from build123d import *

# Parameters (mm, degrees)
F0_R     = 2.45
F0_W     = 1.981159
F0_H     = 1.5
F0_W_2   = 2.842553
F0_W_3   = 1.5
F0_H_2   = 2.468955
F0_W_4   = 2.452735
F0_W_5   = 2.534492
F0_W_6   = 2.289216
F0_H_3   = 2.337886
F0_W_7   = 2.144671
F0_W_8   = 3.006068
F1_DEPTH = 600


with BuildPart() as f1:
    # F0 (on Front) → F1 (new body)
    with BuildSketch(Plane.XZ):
        with BuildLine():
            Line((-53.070132, 53.634533), (-62.125003, 53.634533))
            ThreePointArc((-62.125003, 53.634533), (-64.246324, 52.755854), (-65.125003, 50.634533))
            Line((-65.125003, 50.634533), (-65.125003, 41.826408))
            Line((-65.125003, 41.826408), (-63.625003, 41.826408))
            Line((-63.625003, 41.826408), (-63.625003, 44.295363))
            Line((-63.625003, 44.295363), (-63.625003, 45.603488))
            Line((-63.625003, 45.603488), (-63.625003, 48.301496))
            Line((-63.625003, 48.301496), (-63.625003, 51.134533))
            Line((-63.625003, 51.134533), (-63.625003, 52.134533))
            Line((-63.625003, 52.134533), (-62.625003, 52.134533))
            Line((-62.625003, 52.134533), (-59.837058, 52.134533))
            Line((-59.837058, 52.134533), (-57.975602, 52.134533))
            Line((-57.975602, 52.134533), (-55.912685, 52.134533))
            Line((-55.912685, 52.134533), (-53.070132, 52.134533))
            Line((-53.070132, 52.134533), (-53.070132, 53.634533))
        make_face()
        Polygon((-23.473811, 53.634533), (-46.611269, 53.634533), (-46.611269, 52.134533), (-44.63011, 52.134533), (-41.951072, 52.134533), (-38.108457, 52.134533), (-32.058381, 52.134533), (-27.561702, 52.134533), (-26.479879, 52.134533), (-23.473811, 52.134533), align=None)
        with BuildLine():
            Line((-8.125003, 53.634533), (-17.096702, 53.634533))
            Line((-17.096702, 53.634533), (-17.096702, 52.134533))
            Line((-17.096702, 52.134533), (-14.952031, 52.134533))
            Line((-14.952031, 52.134533), (-12.857073, 52.134533))
            Line((-12.857073, 52.134533), (-10.801355, 52.134533))
            Line((-10.801355, 52.134533), (-7.625003, 52.134533))
            Line((-7.625003, 52.134533), (-6.625003, 52.134533))
            Line((-6.625003, 52.134533), (-6.625003, 51.134533))
            Line((-6.625003, 51.134533), (-6.625003, 48.318361))
            Line((-6.625003, 48.318361), (-6.625003, 46.813633))
            Line((-6.625003, 46.813633), (-6.625003, 44.164294))
            Line((-6.625003, 44.164294), (-6.625003, 41.826408))
            Line((-6.625003, 41.826408), (-5.125003, 41.826408))
            Line((-5.125003, 41.826408), (-5.125003, 50.634533))
            ThreePointArc((-5.125003, 50.634533), (-6.003683, 52.755854), (-8.125003, 53.634533))
        make_face()
        with BuildLine():
            Line((-63.625003, 35.285785), (-65.125003, 35.285785))
            Line((-65.125003, 35.285785), (-65.125003, 26.373664))
            ThreePointArc((-65.125003, 26.373664), (-64.246324, 24.252343), (-62.125003, 23.373664))
            Line((-62.125003, 23.373664), (-53.070132, 23.373664))
            Line((-53.070132, 23.373664), (-53.070132, 24.873664))
            Line((-53.070132, 24.873664), (-55.522867, 24.873664))
            Line((-55.522867, 24.873664), (-57.403297, 24.873664))
            Line((-57.403297, 24.873664), (-59.447241, 24.873664))
            Line((-59.447241, 24.873664), (-62.625003, 24.873664))
            Line((-62.625003, 24.873664), (-63.625003, 24.873664))
            Line((-63.625003, 24.873664), (-63.625003, 25.873664))
            Line((-63.625003, 25.873664), (-63.625003, 29.088415))
            Line((-63.625003, 29.088415), (-63.625003, 31.459391))
            Line((-63.625003, 31.459391), (-63.625003, 33.012789))
            Line((-63.625003, 33.012789), (-63.625003, 35.285785))
        make_face()
        Polygon((-46.611269, 24.873664), (-46.611269, 23.373664), (-23.473811, 23.373664), (-23.473811, 24.873664), (-23.55557, 24.873664), (-26.090062, 24.873664), (-27.806975, 24.873664), (-31.894863, 24.873664), (-38.35373, 24.873664), (-41.787558, 24.873664), (-44.158534, 24.873664), align=None)
        with BuildLine():
            Line((-5.125003, 26.373664), (-5.125003, 35.285785))
            Line((-5.125003, 35.285785), (-6.625003, 35.285785))
            Line((-6.625003, 35.285785), (-6.625003, 32.88172))
            Line((-6.625003, 32.88172), (-6.625003, 30.789106))
            Line((-6.625003, 30.789106), (-6.625003, 29.120862))
            Line((-6.625003, 29.120862), (-6.625003, 25.773664))
            Line((-6.625003, 25.773664), (-6.625003, 24.873664))
            Line((-6.625003, 24.873664), (-7.525003, 24.873664))
            Line((-7.525003, 24.873664), (-10.883111, 24.873664))
            Line((-10.883111, 24.873664), (-13.090572, 24.873664))
            Line((-13.090572, 24.873664), (-14.807486, 24.873664))
            Line((-14.807486, 24.873664), (-17.096702, 24.873664))
            Line((-17.096702, 24.873664), (-17.096702, 23.373664))
            Line((-17.096702, 23.373664), (-8.125003, 23.373664))
            ThreePointArc((-8.125003, 23.373664), (-6.003683, 24.252343), (-5.125003, 26.373664))
        make_face()
        Polygon((-28.238816, 51.493694), (-27.561702, 52.134533), (-32.058381, 52.134533), (-38.108457, 52.134533), (-40.070646, 50.607581), (-40.070646, 47.991332), (-41.133494, 46.110899), (-44.240293, 43.004104), (-45.057871, 41.695979), (-45.057871, 35.891176), (-44.076775, 34.256019), (-40.888221, 30.98571), (-39.988887, 29.10528), (-39.988887, 27.63364), (-39.253068, 26.325515), (-38.35373, 24.873664), (-31.894863, 24.873664), (-27.806975, 24.873664), (-28.624554, 26.259338), (-28.624554, 28.548557), (-23.719084, 33.454025), (-17.178463, 33.454025), (-12.354753, 29.529651), (-12.354753, 26.177581), (-13.090572, 24.873664), (-10.883111, 24.873664), (-10.883111, 29.120862), (-6.625003, 29.120862), (-6.625003, 30.789106), (-10.493293, 30.789106), (-14.581185, 35.285785), (-14.581185, 42.15344), (-9.920991, 46.813633), (-6.625003, 46.813633), (-6.625003, 48.318361), (-10.801355, 48.318361), (-10.801355, 52.134533), (-12.857073, 52.134533), (-11.976291, 51.506915), (-11.976291, 48.246956), (-13.090572, 46.683204), (-17.505493, 43.638769), (-23.21886, 43.638769), (-24.083539, 44.254912), (-28.238816, 48.645393), align=None)
        with Locations((-20.125003, 38.634533)):
            Circle(F0_R, mode=Mode.SUBTRACT)
        Polygon((-57.975602, 48.563634), (-57.975602, 52.134533), (-59.837058, 52.134533), (-59.837058, 48.301496), (-63.625003, 48.301496), (-63.625003, 45.603488), (-62.862098, 46.666339), (-60.082331, 46.666339), (-55.422138, 42.578451), (-55.422138, 35.056733), (-60.000576, 30.478297), (-63.025609, 30.478297), (-63.625003, 31.459391), (-63.625003, 29.088415), (-59.447241, 29.088415), (-59.447241, 24.873664), (-57.403297, 24.873664), (-58.139116, 25.932308), (-58.139116, 28.712073), (-53.397164, 33.454025), (-46.611269, 33.454025), (-41.787558, 29.120862), (-41.787558, 25.687035), (-41.787558, 24.873664), (-38.35373, 24.873664), (-39.253068, 26.325515), (-39.988887, 27.63364), (-39.988887, 29.10528), (-40.888221, 30.98571), (-44.076775, 34.256019), (-45.057871, 35.891176), (-45.057871, 41.695979), (-44.240293, 43.004104), (-41.133494, 46.110899), (-40.070646, 47.991332), (-40.070646, 50.607581), (-38.108457, 52.134533), (-41.951072, 52.134533), (-41.951072, 47.746059), (-46.611269, 43.985196), (-53.642437, 43.985196), align=None)
        with Locations((-50.125003, 38.634533)):
            Circle(F0_R, mode=Mode.SUBTRACT)
        with Locations((-45.620689, 51.384533)):
            Rectangle(F0_W, F0_H)
        with Locations((-54.491408, 51.384533)):
            Rectangle(F0_W_2, F0_H)
        with Locations((-62.875003, 43.060885)):
            Rectangle(F0_W_3, F0_H_2)
        Polygon((-63.625003, 35.383765), (-63.625003, 35.285785), (-63.625003, 33.012789), (-62.125003, 33.012789), (-62.125003, 35.383765), align=None)
        with Locations((-54.296499, 25.623664)):
            Rectangle(F0_W_4, F0_H)
        with Locations((-45.384901, 25.623664)):
            Rectangle(F0_W_4, F0_H)
        with Locations((-24.822816, 25.623664)):
            Rectangle(F0_W_5, F0_H)
        with Locations((-15.952094, 25.623664)):
            Rectangle(F0_W_6, F0_H)
        Polygon((-6.625003, 32.88172), (-6.625003, 35.285785), (-6.625003, 35.383765), (-8.125003, 35.383765), (-8.125003, 32.88172), align=None)
        with Locations((-7.375003, 42.995351)):
            Rectangle(F0_W_3, F0_H_3)
        with Locations((-16.024366, 51.384533)):
            Rectangle(F0_W_7, F0_H)
        with Locations((-24.976845, 51.384533)):
            Rectangle(F0_W_8, F0_H)
    extrude(amount=F1_DEPTH)


solid = f1.part
Input: part model. Units: mm. Frame: model coordinates. Coordinates: 2 decimals unless noted, no trailing zeros.
1. Cut plane A-A, the plane y = -55. Count the separate pieces of the cut face and the enclosed holes in it, plus the area to 3 significant figures.
Checked values:
separate pieces: 1
enclosed holes: 6
area: 1,010 mm2
2. Ray query, line 1 along X through (y, z) = (-138, 50) (3 decimals); line 2 along X through (y, z) = (-489, 42) (3 decimals); line 3 along X through (y, z) = (-91, 26.5) (3 decimals). Return the intervals inside material, ascending.
Checked values:
line 1: x = -65.125 to -63.625, -59.837 to -57.976, -41.951 to -28.239, -11.976 to -10.801, -6.625 to -5.125
line 2: x = -65.125 to -62.125, -55.422 to -14.581, -8.125 to -5.125
line 3: x = -65.125 to -63.625, -59.447 to -58.139, -41.788 to -28.625, -12.355 to -10.883, -6.625 to -5.125
3. Contact query for flat-ended pins moving along their axis: P1, Ø2.5, axis at x = -7, y = -152.5, coming from the -Z side; P2, Ø0.8, axis at y = -200.5, z = 51.5, coming from the +X side. Output: stop coordinate, or through.
Checked values:
P1: stops at z = 23.37
P2: stops at x = -5.16
